```python
from build123d import *

# Parameters (mm, degrees)
SKETCH_196_W        = 95
SKETCH_196_H        = 55
EXTRUDE_2_DEPTH     = 110
SKETCH_556_W        = 89
SKETCH_556_H        = 103
CUT_EXTRUDE_1_DEPTH = 52
SKETCH_4_W          = 10
SKETCH_4_H          = 19
CUT_EXTRUDE_2_DEPTH = 10
SKETCH_5_R          = 2.65
CUT_EXTRUDE_3_DEPTH = 10
SKETCH_6_W          = 20
SKETCH_6_H          = 20
CUT_EXTRUDE_4_DEPTH = 2
CUT_EXTRUDE_4_DRAFT = -10
SKETCH_7_R          = 2.65
CUT_EXTRUDE_5_DEPTH = 5
CUT_EXTRUDE_6_DEPTH = 130


with BuildPart() as part:
    # Sketch 196 → Extrude 2 (new body)
    with BuildSketch(Plane.XY):
        with Locations((9.731535207, -3.335016835)):
            Rectangle(SKETCH_196_W, SKETCH_196_H)
    extrude(amount=-EXTRUDE_2_DEPTH)

    # Sketch 556 → Cut-Extrude 1 (cut)
    with BuildSketch(Plane(origin=(0, 24.164983165, 0), x_dir=(1, 0, 0), z_dir=(0, 1, 0))):
        with Locations((9.731535207, 55.5)):
            Rectangle(SKETCH_556_W, SKETCH_556_H)
    extrude(amount=-CUT_EXTRUDE_1_DEPTH, mode=Mode.SUBTRACT)

    # Sketch 4 → Cut-Extrude 2 (cut)
    with BuildSketch(Plane.XY):
        with Locations((37.231535207, -3.968013468)):
            Rectangle(SKETCH_4_W, SKETCH_4_H)
    extrude(amount=-CUT_EXTRUDE_2_DEPTH, mode=Mode.SUBTRACT)

    # Sketch 5 → Cut-Extrude 3 (cut)
    with BuildSketch(Plane.XY):
        with Locations((37.231535207, -17.468013468)):
            Circle(SKETCH_5_R)
    extrude(amount=-CUT_EXTRUDE_3_DEPTH, mode=Mode.SUBTRACT)


with BuildPart() as cut_extrude_4_tool:
    # Sketch 6 → Cut-Extrude 4 (with draft: the straight prism first)
    with BuildSketch(Plane.XY):
        with Locations((37.231535207, -17.468013468)):
            Rectangle(SKETCH_6_W, SKETCH_6_H)
    extrude(amount=-CUT_EXTRUDE_4_DEPTH)
    # Cut-Extrude 4: the draft: its side faces are tilted about the plane it starts from
    cut_extrude_4_sides = [cut_extrude_4_tool.faces().sort_by_distance(p)[0] for p in [
        (27.231535207, -17.468013468, -1),
        (37.231535207, -27.468013468, -1),
        (47.231535207, -17.468013468, -1),
        (37.231535207, -7.468013468, -1),
    ]]
    draft(cut_extrude_4_sides, Plane.XY, CUT_EXTRUDE_4_DRAFT)


with BuildPart() as part_1:
    add(part.part)

    # Cut-Extrude 4: cut by cut_extrude_4_tool
    add(cut_extrude_4_tool.part, mode=Mode.SUBTRACT)

    # Sketch 7 → Cut-Extrude 5 (cut)
    with BuildSketch(Plane.XZ.offset(30.835016835)):
        with Locations(Location((9.731535207, -55, 0), (0, 0, 270))):
            Circle(SKETCH_7_R)
        with BuildLine():
            Line((-12.711989835, -23.70260728), (32.17506025, -23.70260728))
            ThreePointArc((32.17506025, -23.70260728), (35.675426541, -27.202973571), (32.17506025, -30.703339862))
            Line((32.17506025, -30.703339862), (-12.711989835, -30.703339862))
            ThreePointArc((-12.711989835, -30.703339862), (-16.212356126, -27.202973571), (-12.711989835, -23.70260728))
        make_face()
    extrude(amount=-CUT_EXTRUDE_5_DEPTH, mode=Mode.SUBTRACT)

    # Sketch 8 → Cut-Extrude 6 (cut)
    with BuildSketch(Plane(origin=(0, 0, -110), x_dir=(-1, 0, 0), z_dir=(0, 0, -1))):
        with BuildLine():
            Line((24.415116535, 11.664983165), (24.415116535, -18.335016835))
            ThreePointArc((24.415116535, -18.335016835), (19.056084672, -23.694048698), (13.697052809, -18.335016835))
            Line((13.697052809, -18.335016835), (13.697052809, 11.664983165))
            ThreePointArc((13.697052809, 11.664983165), (19.056084672, 17.024015028), (24.415116535, 11.664983165))
        make_face()
    extrude(amount=-CUT_EXTRUDE_6_DEPTH, mode=Mode.SUBTRACT)


solid = part_1.part
```
Work out the finished part from the listing and answer in its coordinate system (mm). A direction names the side the tool comes from. Round coordinates to 2 decimals unless told otherwise and drop trailing zeros. Loops run counter-clockwise (first coordinate to the right, second up) from the corner with the lowest first, then second, coordinate; pieces in that order, holes last. Notation, with made-up numbers: (-12.75, -39.5) -> (-5.75, -39.5) arc R27 cw to (-5.75, -4.5) -> close; hole circle Ø1 at (-4.75, -35.5). An arc over 180 degrees is marked (long way). Write each question's results on one line, items separated by ' | '. Start each with the question number.
1. Section A-A (z = -55) is taken. Determine the outline of the cut face in (x, y).
2. A tool of negligible diameter and unlimited length cuts with its end or side. For faces 1 (the face through (34.584, -17.351, -2.986)), 2 (the face through (-24.415, -3, -2)), 3 (the face through (35.675, -29.356, -27.126)), 4 (the face through (9, -1, -4)), from which of +Z, -Z, +X, -X, +Y, -Y can it reach the whole face along a straight path? Write none if from no direction.
3. Section D-D (y = -4) is taken. Determine the outline of the cut face in (x, z).
4. Section B-B (x = -0.5) is taken. Determine the outline of the cut face in (y, z).
5. Given pin 1 Ø8 at (x, y) = (33, 7.5) entering from +Z; pin 2 Ø1 at (x, z) = (43.5, -59.5) entering from +Y (3 decimals); pin 3 Ø5 at (x, z) = (9.73, -55) entering from -Y, each flat-ended and moving along its own axis, determine where each tip first touches the part or whether it passes through.
6. Find the intervals of material crossed by probe 1 along X at (y, z) = (-24, -47); probe 2 along Z at (x, y) = (41.5, 8); probe 3 along X at (y, z) = (-29.8, -55), in increasing order. Write a range as from..to.
7. For a pull along Z with two mould halves and no side action, classify faces 5 (the face through (37, 5.532, -2)), 6 (the face through (19, -27.835, -56)), 7 (the face through (35, -19.5, -2)) as +Z half, -Z half, draft (parallel to the pull), parting line (faces both ways), or undercut.
8. Section C-C (y = 8.5) is taken. Determine the outline of the cut face in (x, z), plus the area to 3 significant figures.
Evaluation:
1) outline: (-37.77, -30.84) -> (7.08, -30.84) -> (7.08, -27.84) -> (-34.77, -27.84) -> (-34.77, 24.16) -> (-37.77, 24.16) -> close; (12.38, -30.84) -> (57.23, -30.84) -> (57.23, 24.16) -> (54.23, 24.16) -> (54.23, -27.84) -> (12.38, -27.84) -> close
2) face 1: +Z | face 2: +Z, -Z | face 3: +Y, -Y | face 4: +Y
3) outline: (-37.77, -110) -> (-24.42, -110) -> (-24.42, -107) -> (-34.77, -107) -> (-34.77, -4) -> (-24.42, -4) -> (-24.42, 0) -> (-37.77, 0) -> close; (-13.7, -110) -> (57.23, -110) -> (57.23, 0) -> (42.23, 0) -> (42.23, -4) -> (54.23, -4) -> (54.23, -107) -> (-13.7, -107) -> close; (-13.7, -4) -> (32.23, -4) -> (32.23, 0) -> (-13.7, 0) -> close
4) outline: (-30.84, -110) -> (24.16, -110) -> (24.16, -107) -> (-27.84, -107) -> (-27.84, -30.7) -> (-30.84, -30.7) -> close; (-30.84, -23.7) -> (-27.84, -23.7) -> (-27.84, -4) -> (24.16, -4) -> (24.16, 0) -> (-30.84, 0) -> close
5) pin 1: stops at z = 0 | pin 2: stops at y = -27.835 | pin 3: passes through
6) probe 1: x = -37.77..-34.77, 54.23..57.23 | probe 2: z = -110..-107, -4..0 | probe 3: x = -37.77..7.08, 12.38..57.23
7) face 5: draft | face 6: undercut | face 7: +Z half
8) outline: (-37.77, -110) -> (-24.42, -110) -> (-24.42, -107) -> (-34.77, -107) -> (-34.77, -4) -> (-24.42, -4) -> (-24.42, 0) -> (-37.77, 0) -> close; (-13.7, -110) -> (57.23, -110) -> (57.23, 0) -> (-13.7, 0) -> (-13.7, -4) -> (54.23, -4) -> (54.23, -107) -> (-13.7, -107) -> close | area: 1,210 mm2
